Work out the finished part from the listing and answer in its coordinate system (mm). A direction names the side the tool comes from. Give positions to 0.01 mm unless a question says otherwise; leave off trailing zeros. Loops run counter-clockwise (first coordinate to the right, second up) from the corner with the lowest first, then second, coordinate; pieces in that order, holes last. Notation, with made-up numbers: M 34,40 L 93,40 A30 cw 93,76 Z; hole C 1,74.5 d4. An arc over 180 degrees is marked long. Write item = value, one per line. Start each with the question number.
1. Flat-ended cylindrical pins translate along their axes: pin 1 Ø3 at (y, z) = (-0.5, -17) entering from +X; pin 2 Ø5 at (y, z) = (0.5, -20) entering from -X; pin 3 Ø5 at (y, z) = (-10.5, -21) entering from -X. Find the tip coordinate at first contact, or state that the pin passes through.
2. The mould has two halves that part along X. Classify faces 1 (the face through (0.35, -0.11, -11.36)), 2 (the face through (-4, 13, -6)), 3 (the face through (-4.9, -8, -20.1)): released by +X, released by -X, zero draft, split by the parting line, or undercut.
3. Consider L1, parallel to Y at x = 0, z = -22.5; L2, parallel to Z at x = -8, y = 6; L3, parallel to X at y = 3, z = 0. Determine where each line is inside the solid, lowest interval first. Write a range as [from, to].
4. Section A-A on x = -14.5 is taken. Determine the outline of the cut face in (y, z), plus the area to 3 significant figures.
5. For faces 4 (the face through (-7, 0, -20)), 5 (the face through (5, -7.9, -20.1)), 6 (the face through (0.28, -10.95, -3.45)), 7 (the face through (-1.409, 4.888, -6.345)), determine the directions among +Z, -Z, +X, -X, +Y, -Y from which every point of the face is accessible in a straight line to the end or side of a thin tool.
6. Section C-C on y = -9.5 is taken. Determine the outline of the cut face in (x, z).
7. Section D-D on y = 6 is taken. Determine the outline of the cut face in (x, z), plus the area to 3 significant figures.
```python
from build123d import *

# Parameters (mm, degrees)
F1_DEPTH  = 20
F2_W      = 14
F2_H      = 20
F3_DEPTH  = 14
F4_R      = 6.99999
F6_D      = 13
F6_DEPTH  = 16
F6_TIP    = 3.9055940237
F7_R      = 2
F8_DEPTH  = 20
F10_D     = 4.2
F10_DEPTH = 14.6
F10_TIP   = 1.2618073


# Not quite as in the source:
# - a fillet or chamfer is up to 0.001 mm smaller than in the source, because OpenCascade refuses the exact size


with BuildPart() as f1:
    # F0 (on Right) → F1 (new body, symmetric)
    with BuildSketch(Plane.YZ):
        Polygon((-13, -13), (13, -13), (13, 13), (-13, 13), (-13, 7), (-8.9585481157, 0), (-13, -7), align=None)
    extrude(amount=F1_DEPTH, both=True)

    # F2 (on face) → F3 (join)
    with BuildSketch(Plane(origin=(0, 0, -13), x_dir=(1, 0, 0), z_dir=(0, 0, -1))):
        Rectangle(F2_W, F2_H)
    extrude(amount=F3_DEPTH)

    # F4 (radius 7 in the source; OpenCascade refuses exactly that, so slightly less here)
    f4_edges = [f1.edges().sort_by_distance(p)[0] for p in [
        (7, -10, -20),
        (-7, -10, -20),
        (7, 10, -20),
        (-7, 10, -20),
    ]]
    fillet(f4_edges, radius=F4_R)

    # F6
    with Locations(Plane(origin=(0, 13, 0), x_dir=(-1, 0, 0), z_dir=(0, 1, 0))):
        with Locations((0, 0)):
            Hole(F6_D / 2, depth=F6_DEPTH)
            with Locations((0, 0, -(F6_DEPTH + F6_TIP / 2))):  # 118° drill point
                Cone(0, F6_D / 2, F6_TIP, mode=Mode.SUBTRACT)

    # F7 (on Right) → F8 (cut, symmetric)
    with BuildSketch(Plane.YZ):
        with Locations((6, 6.5)):
            Circle(F7_R)
    extrude(amount=F8_DEPTH, both=True, mode=Mode.SUBTRACT)

    # F10
    with Locations(Plane(origin=(0, 0, -27), x_dir=(1, 0, 0), z_dir=(0, 0, -1))):
        with Locations((0, 0)):
            Hole(F10_D / 2, depth=F10_DEPTH)
            with Locations((0, 0, -(F10_DEPTH + F10_TIP / 2))):  # 118° drill point
                Cone(0, F10_D / 2, F10_TIP, mode=Mode.SUBTRACT)


solid = f1.part
```
Verdict:
q1.pin_1 = 7
q1.pin_2 = -7
q1.pin_3 = -4.9
q2.face_1 = undercut
q2.face_2 = zero draft
q2.face_3 = released by -X
q3.L1 = [-10, -2.1], [2.1, 10]
q3.L2 = [-13, 4.5], [8.5, 13]
q3.L3 = [-20, -6.5], [6.5, 20]
q4.outline = M -13,-13 L 13,-13 L 13,13 L -13,13 L -13,7 L -8.96,0 L -13,-7 Z; hole C 6,6.5 d4
q4.area = 635 mm2
q5.face_4 = -Z, -X, +Y, -Y
q5.face_5 = -Z, +X, -Y
q5.face_6 = +X, -X, -Y
q5.face_7 = +Y
q6.outline = M -20,-13 L -2.6,-13 L -2.6,-27 L 2.6,-27 L 2.6,-13 L 20,-13 L 20,-0.94 L -20,-0.94 Z; M -20,0.94 L 20,0.94 L 20,13 L -20,13 Z
q7.outline = M -20,-13 L -6.32,-13 L -6.32,-27 L 6.32,-27 L 6.32,-13 L 20,-13 L 20,4.5 L 4.69,4.5 A6.5 cw long -4.69,4.5 L -20,4.5 Z; M -20,8.5 L 20,8.5 L 20,13 L -20,13 Z
q7.area = 937 mm2
